Here's how the part is built. I have some questions about the finished solid (model axes, mm). Face numbers are marked on the shaded views. A direction names the side the tool comes from. Round coordinates to 2 decimals unless told otherwise and drop trailing zeros. Write each loop counter-clockwise with the first axis right and the second up, starting at its lowest first coordinate (ties: lowest second). Pieces come first, ordered by that corner, then holes. Notation, with made-up numbers: (84, 10) -> (100, 10) arc R19 cw to (100, 24) -> close; hole circle Ø10 at (35, -36.75). An arc over 180 degrees is marked (long way). Answer as CSV lines item,"result".
Autodesk Inventor part; units mm, degrees
ref_plane "YZ Plane" through (0, 0, 0) normal (1, 0, 0) x (0, 1, 0)
ref_plane "XZ Plane" through (0, 0, 0) normal (0, 1, 0) x (-1, 0, 0)
ref_plane "XY Plane" through (0, 0, 0) normal (0, 0, 1) x (1, 0, 0)
sketch "Sketch1" plane through (0, 0, 0) normal (1, 0, 0) x (0, 1, 0)
  line L0 (0, 5.2) -> (0, -3.9)
  line L1 (0, -3.9) -> (1.3, -3.9)
  line L2 (1.3, -3.9) -> (6, 0.8)
  line L3 (6, 0.8) -> (6, 5.2)
  line L4 (6, 5.2) -> (0, 5.2)
  point P0 (0, 0)
  dimension "d0" = 9.1
  dimension "d1" = 6
  dimension "d2" = 0
  dimension "d3" = 5.2
  dimension "d4" = 1.3
  dimension "d5" = 45
extrude "Extrusion1" add sketch "Sketch1" along normal mid plane 6
sketch "Sketch2" plane through (-3, 0, 5.2) normal (0, 0, 1) x (1, 0, 0)
  circle A0 centre (3, 3) radius 2.4
  point P0 (3, 0)
  dimension "d8" = 4.8
extrude "Extrusion2" add sketch "Sketch2" along normal blind 3.2
fillet "Fillet1" radius 2.4 1 edges at (-2.4, 3, 8.4)
sketch "Sketch3" plane through (-3, 0, -3.9) normal (0, -1, 0) x (1, 0, 0)
  circle A0 centre (1.73, 3.9) radius 0.25
  circle A1 centre (4.27, 3.9) radius 0.25
  point P0 (3, 3.9)
  dimension "d12" = 0.5
  dimension "d13" = 0.5
  dimension "d14" = 2.54
  dimension "d15" = 1.27
  dimension "d16" = 0
  dimension "d17" = 0
extrude "Extrusion3" add sketch "Sketch3" along normal blind 3.8
properties part number "Multicomp-2118128"
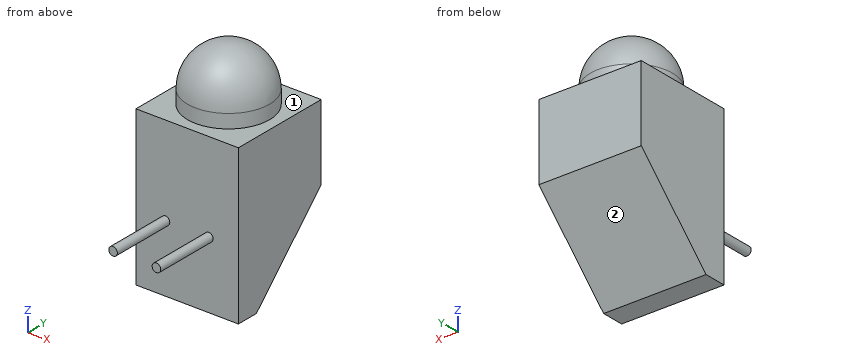
1. If I drill on line 1 (Z direction, x = 1.6, y = 0.5); line 2 (Y direction, x = 1.8, z = 3); line 3 (Y direction, x = -0.4, z = 0), over which ranges is the centre line in solid material (lowest first)?
Numbers:
line 1,"z = -3.9 to 5.2"
line 2,"y = 0 to 6"
line 3,"y = 0 to 5.2"
2. Suppose I cut it at C-C on y = 3. Please give me the cut outline in (x, z).
Numbers:
outline,"(-3, -2.2) -> (3, -2.2) -> (3, 5.2) -> (2.4, 5.2) -> (2.4, 6) arc R2.4 ccw to (-2.4, 6) -> (-2.4, 5.2) -> (-3, 5.2) -> close"
3. Suppose I cut it at A-A on z = 0. Please give me the cut outline in (x, y), and give its area (3 significant figures).
Numbers:
outline,"(-3, 0) -> (-1.52, 0) -> (-1.52, -3.8) -> (-1.02, -3.8) -> (-1.02, 0) -> (1.02, 0) -> (1.02, -3.8) -> (1.52, -3.8) -> (1.52, 0) -> (3, 0) -> (3, 5.2) -> (-3, 5.2) -> close"
area,"35.0 mm^2"
4. Suppose I cut it at D-D on y = -2.75. Please give me the cut outline in (x, z).
Numbers:
outline,"circle Ø0.5 at (-1.27, 0); circle Ø0.5 at (1.27, 0)"
5. Suppose I cut it at B-B on x = 0. Please give me the cut outline in (y, z).
Numbers:
outline,"(0, -3.9) -> (1.3, -3.9) -> (6, 0.8) -> (6, 5.2) -> (5.4, 5.2) -> (5.4, 6) arc R2.4 ccw to (0.6, 6) -> (0.6, 5.2) -> (0, 5.2) -> close"
6. For pin 1 Ø1.5 at (x, y) = (2.5, -0.5) entering from +Z; pin 2 Ø3 at (x, y) = (-0.5, -2.5) entering from -Z, each with a flat end and sliding along its axis, tell me the tip position at first contact or that it passes through.
Numbers:
pin 1,"stops at z = 5.2"
pin 2,"stops at z = -0.25"
7. On a 3-axis mill with a long thin cutter (end or side, diameter ignored), from which of +Z, -Z, +X, -X, +Y, -Y can I reach the whole of each face in a straight line? I mean the marked faces 1 and 2. Say none if no direction works.
Numbers:
face 1,"+Z"
face 2,"-Z, +X, -X, +Y"
